Verification items for the finished model (mm, model axes). A direction names the side the tool comes from. Give positions to 0.01 mm unless a question says otherwise; leave off trailing zeros. Write each loop counter-clockwise with the first axis right and the second up, starting at its lowest first coordinate (ties: lowest second). Pieces come first, ordered by that corner, then holes. Notation, with made-up numbers: (73.5, 86.5) -> (114.5, 86.5) arc R20 cw to (114.5, 97.5) -> close; hole circle Ø9 at (76, 18.25). An arc over 180 degrees is marked (long way). Answer as CSV lines item,"result".
```python
from build123d import *

# Parameters (mm, degrees)
BOSS_EXTRUDE1_DEPTH      = 16
SKETCH2_W                = 1
SKETCH2_H                = 5
CUT_EXTRUDE1_DEPTH       = 24.706539182
FILLET1_R                = 0.5
CIRPATTERN1_COUNT        = 8
FILLET1_OF_CIRPATTERN1_R = 0.5
CUT_EXTRUDE2_DEPTH       = 24.706539182
CUT_EXTRUDE3_DEPTH       = 24.900836805
CUT_EXTRUDE3_DEPTH_BACK  = 24.900836805
SKETCH5_R                = 0.80645
SKETCH5_R_2              = 0.825
FILLET2_R                = 1
FILLET3_R                = 3
CUT_EXTRUDE5_DEPTH       = 10


# Some blends are built 0.0001 mm under size
with BuildPart() as part:
    # Sketch1 → Boss-Extrude1 (new body)
    with BuildSketch(Plane(origin=(0, 0, 0), x_dir=(1, 0, 0), z_dir=(0, 1, 0))):
        with BuildLine():
            Line((-3.98274298, -0.525180459), (-15, -1.25))
            Line((-15, -1.25), (-15, -4))
            Line((-15, -4), (-8.062257748, -4))
            ThreePointArc((-8.062257748, -4), (0.804756356, -8.963948193), (8.645808233, -2.5))
            Line((8.645808233, -2.5), (13, -2.5))
            Line((13, -2.5), (13, 2.5))
            Line((13, 2.5), (8.645808233, 2.5))
            ThreePointArc((8.645808233, 2.5), (0.804756356, 8.963948193), (-8.062257748, 4))
            Line((-8.062257748, 4), (-15, 4))
            Line((-15, 4), (-15, 1.25))
            Line((-15, 1.25), (-3.98274298, 0.525180459))
            ThreePointArc((-3.98274298, 0.525180459), (0.27121874, 4.25396172), (4, 0))
            ThreePointArc((4, 0), (0.27121874, -4.25396172), (-3.98274298, -0.525180459))
        make_face()
    extrude(amount=BOSS_EXTRUDE1_DEPTH)

    # Sketch2 → Cut-Extrude1 (cut, through all)
    with BuildSketch(Plane(origin=(0, 16, 0), x_dir=(1, 0, 0), z_dir=(0, 1, 0))):
        with Locations((0, 3.5)):
            Rectangle(SKETCH2_W, SKETCH2_H)
    cut_extrude1 = extrude(amount=-CUT_EXTRUDE1_DEPTH, mode=Mode.SUBTRACT)

    # Fillet1
    fillet1_edges = [part.edges().sort_by_distance(p)[0] for p in [
        (-0.5, 8, -6),
        (0.5, 8, -6),
    ]]
    fillet(fillet1_edges, radius=FILLET1_R - 0.0001)  # a hair under: the kernel refuses the full size

    # CirPattern1: Cut-Extrude1 ×8 about axis, 2 skipped
    cirpattern1_axis = Axis((0, 0, 0), (0, -1, 0))
    add([cut_extrude1.rotate(cirpattern1_axis, i * 360 / CIRPATTERN1_COUNT) for i in range(1, CIRPATTERN1_COUNT) if i not in (2, 6)], mode=Mode.SUBTRACT)

    # Fillet1 of CirPattern1
    fillet1_of_cirpattern1_edges = [part.edges().sort_by_distance(p)[0] for p in [
        (3.889087297, 8, -4.596194078),
        (4.596194078, 8, -3.889087297),
        (4.596194078, 8, 3.889087297),
        (3.889087297, 8, 4.596194078),
        (0.5, 8, 6),
        (-0.5, 8, 6),
        (-3.889087297, 8, 4.596194078),
        (-4.596194078, 8, 3.889087297),
        (-4.596194078, 8, -3.889087297),
        (-3.889087297, 8, -4.596194078),
    ]]
    fillet(fillet1_of_cirpattern1_edges, radius=FILLET1_OF_CIRPATTERN1_R - 0.0001)  # a hair under: the kernel refuses the full size

    # Sketch4 → Cut-Extrude2 (cut, through all)
    with BuildSketch(Plane(origin=(0, 16, 0), x_dir=(1, 0, 0), z_dir=(0, 1, 0))):
        Polygon((7.75, -0.5), (7.75, 0.5), (13, 0.5), (13, -0.5), (13, -2.5), (7.75, -2.5), align=None)
    extrude(amount=-CUT_EXTRUDE2_DEPTH, mode=Mode.SUBTRACT)

    # Sketch5 → Cut-Extrude3 (cut, two sides: drawn at the far end of the back side and taken through both)
    with BuildSketch(Plane.XY.offset(-0.5).offset(-CUT_EXTRUDE3_DEPTH_BACK)):
        with Locations((10.5, 13)):
            Circle(SKETCH5_R)
        with Locations((10.5, 3)):
            Circle(SKETCH5_R)
        with Locations((-12.5, 13)):
            Circle(SKETCH5_R_2)
        with Locations((-12.5, 3)):
            Circle(SKETCH5_R_2)
    extrude(amount=CUT_EXTRUDE3_DEPTH + CUT_EXTRUDE3_DEPTH_BACK, mode=Mode.SUBTRACT)

    # Fillet2
    fillet2_edges = [part.edges().sort_by_distance(p)[0] for p in [
        (-3.98274298, 8, -0.525180459),
        (-15, 8, -1.25),
        (-15, 8, -4),
        (13, 8, -2.5),
        (-15, 8, 4),
        (-15, 8, 1.25),
        (-3.98274298, 8, 0.525180459),
    ]]
    fillet(fillet2_edges, radius=FILLET2_R)

    # Fillet3
    # the kernel refuses this fillet: 3 mm, written as the material it adds along each edge
    with BuildSketch(Plane(origin=(-8.062257748, 0, -4), x_dir=(-1, 0, 0), z_dir=(0, 1, 0))) as fillet3_piece_1:
        with BuildLine():
            CenterArc((1.684536597, -3), FILLET3_R, 90, 54.314665287)
            ThreePointArc((-0.75216199, -1.25), (-0.350711983, -0.640265285), (0, 0))
            Line((0, 0), (1.684536597, 0))
        make_face()
    extrude(amount=16)
    with BuildSketch(Plane(origin=(8.645808233, 0, -2.5), x_dir=(-0.36980540281703944, 0, -0.9291092314939762), z_dir=(0, 1, 0))) as fillet3_piece_2_section:
        with BuildLine():
            CenterArc((2.040484874, -2.985804583), FILLET3_R, 95.575996261, 62.720387264)
            Line((-0.74684282, -1.876388375), (0, 0))
            ThreePointArc((0, 0), (0.874493518, -0.04258625), (1.748987035, 0))
        make_face()
    fillet3_piece_2 = extrude(amount=16, mode=Mode.PRIVATE)
    fillet3_piece_2 = fillet3_piece_2 - Plane(origin=(10.5, 13, -2.86106774), x_dir=(1, 0, 0), z_dir=(0, 0, 1)) * Cylinder(0.80645, 40, mode=Mode.PRIVATE)
    fillet3_piece_2 = fillet3_piece_2 - Plane(origin=(10.5, 3, -2.86106774), x_dir=(1, 0, 0), z_dir=(0, 0, 1)) * Cylinder(0.80645, 40, mode=Mode.PRIVATE)
    add(fillet3_piece_2)
    with BuildSketch(Plane(origin=(-8.062257748, 0, 4), x_dir=(0.5155850316607751, 0, 0.8568384183306427), z_dir=(0, 1, 0))) as fillet3_piece_3:
        with BuildLine():
            CenterArc((1.701993401, -2.990130768), FILLET3_R, 94.648767376, 54.314665287)
            Line((-0.868521854, -1.443375673), (0, 0))
            ThreePointArc((0, 0), (0.729425743, -0.029607696), (1.458851486, 0))
        make_face()
    extrude(amount=16)

    # Sketch7 → Cut-Extrude5 (cut)
    with BuildSketch(Plane(origin=(0, 0, -2.5), x_dir=(-1, 0, 0), z_dir=(0, 0, -1))):
        Polygon((-10.5, 15.367136104), (-12.55, 14.183568052), (-12.55, 11.816431948), (-10.5, 10.632863896), (-8.45, 11.816431948), (-8.45, 14.183568052), align=None)
        Polygon((-10.5, 5.367136104), (-12.55, 4.183568052), (-12.55, 1.816431948), (-10.5, 0.632863896), (-8.45, 1.816431948), (-8.45, 4.183568052), align=None)
    extrude(amount=CUT_EXTRUDE5_DEPTH, mode=Mode.SUBTRACT)


solid = part.part
```
1) Scan lines: line 1 along Y through (x, z) = (-12.5, -2.3) (3 decimals); line 2 along Z through (x, y) = (4.25, 13); line 3 along X through (y, z) = (3, 2.9) (3 decimals). Record each from-to range of solid material in increasing order.
Reported:
line 1,"0 to 2.175, 3.825 to 12.175, 13.825 to 16"
line 2,"-7.93 to -4.24, -3.54 to 3.54, 4.24 to 7.93"
line 3,"-15 to -13.325, -11.675 to -3.607, 3.607 to 8.52"
2) Draft check along Y on faces 1 (the flat face through (-1, 0, -5)), 2 (the flat face through (-0.5, 8, -5)), 3 (the cylindrical face through (-13.155, 2.498, 2.495)). Enter one of: +Y half, -Y half, draft (parallel to the pull), parting line (faces both ways), or undercut.
Reported:
face 1,"-Y half"
face 2,"draft"
face 3,"undercut"
3) Section check B-B (x = -7.75). Record the boundary of the cut face in (y, z).
Reported:
outline,"(0, -4.76) -> (16, -4.76) -> (16, -0.77) -> (0, -0.77) -> close; (0, 0.77) -> (16, 0.77) -> (16, 4.76) -> (0, 4.76) -> close"
4) Section check D-D (y = 13). State how many separate pieces and enclosed holes the cut face has, and give its area (3 significant figures).
Reported:
separate pieces,"4"
enclosed holes,"0"
area,"212 mm²"
5) Tool access check on faces 4 (the flat face through (-12, 8, 4)), 5 (the flat face through (10, 8, -0.5)), 6 (the flat face through (8.45, 3, -3)), 7 (the flat face through (0.5, 8, -5)), 8 (the flat face through (-12, 8, -4)). Record the directions out of +Z, -Z, +X, -X, +Y, -Y that give a thin tool (end or side, any length) a straight path to the whole face; none if there is none.
Reported:
face 4,"+Z, -X, +Y, -Y"
face 5,"+X, +Y, -Y"
face 6,"-Z, +X"
face 7,"+Y, -Y"
face 8,"-Z, -X, +Y, -Y"
6) Depth check by flat-ended pin: pin 1 (1 mm diameter, centred on y = 10, z = 4.5, fed in from +X); pin 2 (1.9 mm diameter, centred on x = -12.5, y = 13, fed in from -Z); pin 3 (8 mm diameter, centred on x = -6, y = 5.5, fed in from -Z); pin 4 (8 mm diameter, centred on y = 10.5, z = 3.5, fed in from -X). Enter the tip coordinate at first touch or a pass-through.
Reported:
pin 1,"x = 8.06"
pin 2,"z = -4"
pin 3,"z = -8.77"
pin 4,"x = -15"
7) Section check A-A (x = -12.5). Record the boundary of the cut face in (y, z) (3 decimals).
Reported:
outline,"(0, -4) -> (2.175, -4) -> (2.175, -1.086) -> (0, -1.086) -> close; (0, 1.086) -> (2.175, 1.086) -> (2.175, 4) -> (0, 4) -> close; (3.825, -4) -> (12.175, -4) -> (12.175, -1.086) -> (3.825, -1.086) -> close; (3.825, 1.086) -> (12.175, 1.086) -> (12.175, 4) -> (3.825, 4) -> close; (13.825, -4) -> (16, -4) -> (16, -1.086) -> (13.825, -1.086) -> close; (13.825, 1.086) -> (16, 1.086) -> (16, 4) -> (13.825, 4) -> close"
8) Section check C-C (x = 11). Record the boundary of the cut face in (y, z), and give its area (3 significant figures).
Reported:
outline,"(0, -2.5) -> (2.37, -2.5) -> (2.37, -0.5) -> (0, -0.5) -> close; (3.63, -2.5) -> (12.37, -2.5) -> (12.37, -0.5) -> (3.63, -0.5) -> close; (13.63, -2.5) -> (16, -2.5) -> (16, -0.5) -> (13.63, -0.5) -> close"
area,"26.9 mm²"
